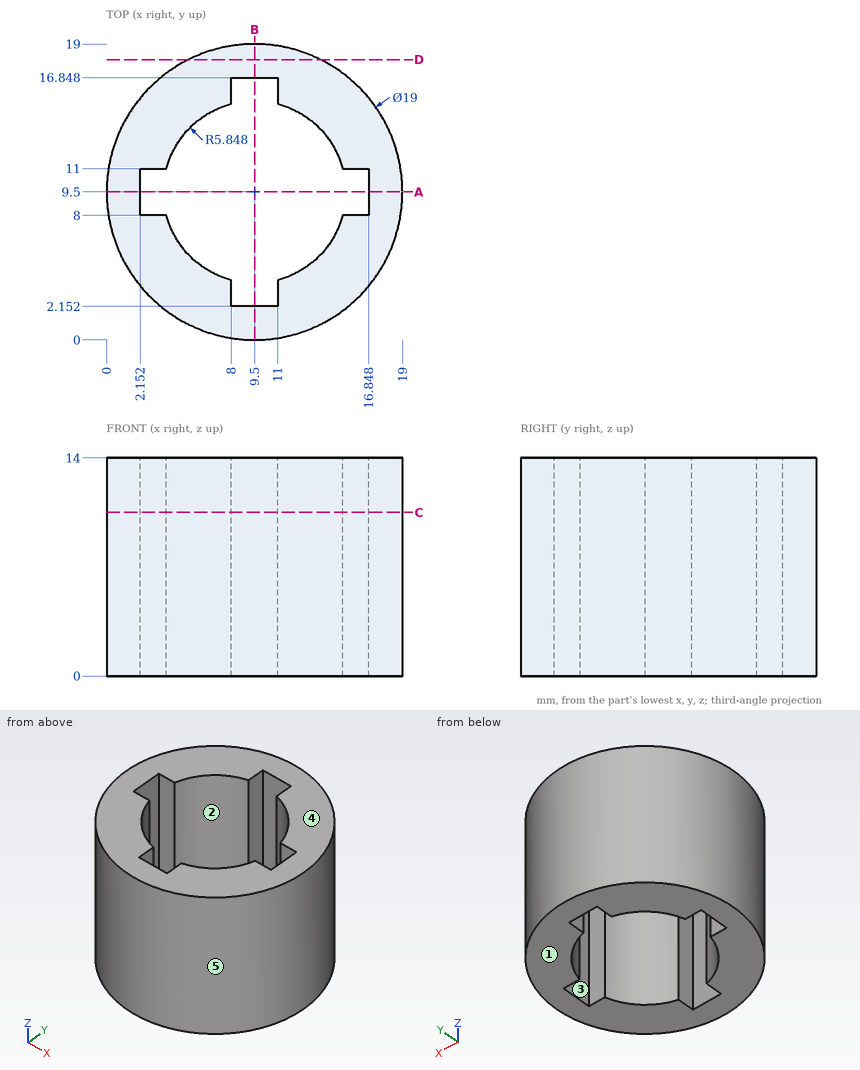
Here's the drawing with two shaded views (mm, measured from the low corner). I have some questions. A direction names the side the tool comes from. Coordinates: 2 decimals unless noted, no trailing zeros. Order: outer loops, then holes, each group sorted by start corner. A loop starts at its lowest first (then second) coordinate and runs counter-clockwise, first axis right, second up. Notation, with made-up numbers: M 60,41 L 89,41 A23 cw 89,64 Z; hole C 16,52 d8. An arc over 180 degrees is marked long. Write item = value, one per line.
(1) For the marked faces 1 and 2, which set-ups out of +Z, -Z, +X, -X, +Y, -Y let a thin tool reach every point of the face, with its end or its side?
Results are:
face_1 = -Z, +X, -X, +Y, -Y
face_2 = +Z, -Z
(2) Suppose I cut it at C-C on z = 10.5. Please give me the cut outline in (x, y), plus the area to 3 significant figures.
Results are:
outline = C 9.5,9.5 d19; hole M 2.15,8 L 3.85,8 A5.85 ccw 8,3.85 L 8,2.15 L 11,2.15 L 11,3.85 A5.85 ccw 15.15,8 L 16.85,8 L 16.85,11 L 15.15,11 A5.85 ccw 11,15.15 L 11,16.85 L 8,16.85 L 8,15.15 A5.85 ccw 3.85,11 L 2.15,11 Z
area = 157 mm2
(3) Suppose I cut it at A-A on y = 9.5. Please give me the cut outline in (x, z).
Results are:
outline = M 0,0 L 2.15,0 L 2.15,14 L 0,14 Z; M 16.85,0 L 19,0 L 19,14 L 16.85,14 Z
(4) For pin 1 Ø4 at (y, z) = (2.5, 12) entering from +X; pin 2 Ø1.9 at (x, z) = (3, 9) entering from +Y; pin 3 Ø5 at (x, z) = (15.5, 5) entering from -Y, each with a flat end and sliding along its axis, tell me the tip position at first contact or that it passes through.
Results are:
pin_1 = 17.58
pin_2 = 17.21
pin_3 = 0.67
(5) I need wall thicknesses on line 1 along Y through (x, z) = (9.5, 6); line 2 along Y through (x, z) = (14.5, 0.5) (1 decimal); line 3 along X through (y, z) = (5.75, 4). Which ranges of each line are inside material? Lowest first, please. Write a range as [from, to].
Results are:
line_1 = [0, 2.15], [16.85, 19]
line_2 = [1.4, 6.5], [12.5, 17.6]
line_3 = [0.77, 5.01], [13.99, 18.23]
(6) Suppose I cut it at D-D on y = 18. Please give me the cut outline in (x, z), plus the area to 3 significant figures.
Results are:
outline = M 5.26,0 L 13.74,0 L 13.74,14 L 5.26,14 Z
area = 119 mm2
(7) If we mould it in two halves opening along Y, with no side actions, what happens to the marked faces 3, 4 and 5? For each: pulls with the +Y half, pulls with the -Y half, needs draft (parallel to the pull), parting line crosses it, or undercut.
Results are:
face_3 = undercut
face_4 = needs draft
face_5 = parting line crosses it
